Geometry check sheet. Reference: drawing and pictorial views, mm from the part's lowest x, y, z. A direction names the side the tool comes from. Round coordinates to 2 decimals unless told otherwise and drop trailing zeros. Write each loop counter-clockwise with the first axis right and the second up, starting at its lowest first coordinate (ties: lowest second). Pieces come first, ordered by that corner, then holes. Notation, with made-up numbers: M 20,34 L 69,34 A20 cw 69,42 Z; hole C 15.25,86 d1. An arc over 180 degrees is marked long. Use a Markdown table: item, result. Add a question column.
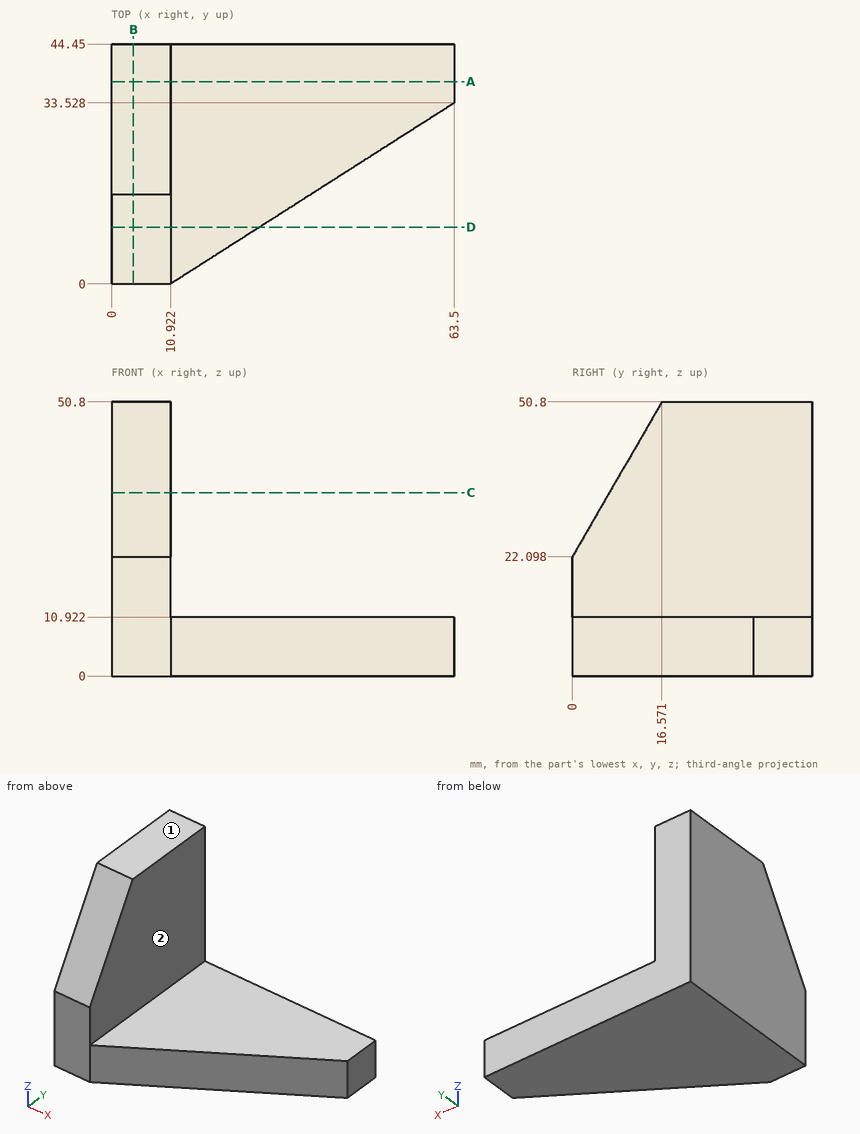
1. Cross-section at B-B on x = 4. Enter the section's corners in (y, z), plus the area to 3 significant figures.
2. Scan lines: line 1 along Z through (x, y) = (30.5, 36); line 2 along Z through (x, y) = (9, 8) (1 decimal). Record each from-to range of solid material in increasing order. Write a range as from..to.
3. Cross-section at A-A on y = 37.5. Enter the section's corners in (x, z), plus the area to 3 significant figures.
4. Cross-section at D-D on y = 10.5. Enter the section's corners in (x, z), plus the area to 3 significant figures.
5. Cross-section at C-C on z = 34. Enter the section's corners in (x, y), plus the area to 3 significant figures.
6. Depth check by flat-ended pin: pin 1 Ø2 at (y, z) = (36, 17) entering from -X; pin 2 Ø4 at (y, z) = (26.5, 29.5) entering from +X; pin 3 Ø8 at (x, y) = (26, 31.5) entering from +Z. Enter the tip coordinate at first touch or a pass-through.
7. Access from +Z, -Z, +X, -X, +Y, -Y to the whole of each face (thin tool, end or side, straight path). Record for the marked faces 1 and 2.
Answer:
| question | item | result |
|---|---|---|
| 1 | outline | M 0,0 L 44.45,0 L 44.45,50.8 L 16.57,50.8 L 0,22.1 Z |
| 1 | area | 2,020 mm^2 |
| 2 | line 1 | z = 0..10.92 |
| 2 | line 2 | z = 0..36 |
| 3 | outline | M 0,0 L 63.5,0 L 63.5,10.92 L 10.92,10.92 L 10.92,50.8 L 0,50.8 Z |
| 3 | area | 1,130 mm^2 |
| 4 | outline | M 0,0 L 27.39,0 L 27.39,10.92 L 10.92,10.92 L 10.92,40.28 L 0,40.28 Z |
| 4 | area | 620 mm^2 |
| 5 | outline | M 0,6.87 L 10.92,6.87 L 10.92,44.45 L 0,44.45 Z |
| 5 | area | 410 mm^2 |
| 6 | pin 1 | stops at x = 0 |
| 6 | pin 2 | stops at x = 10.92 |
| 6 | pin 3 | stops at z = 10.92 |
| 7 | face 1 | +Z, +X, -X, +Y, -Y |
| 7 | face 2 | +Z, +X, +Y, -Y |
